from build123d import *

# Parameters (mm, degrees)
SKETCH_1_W          = 19.8
SKETCH_1_H          = 10.2
EXTRUDE_1_DEPTH     = 6.4
SKETCH_2_R          = 1.175
CUT_EXTRUDE_1_DEPTH = 7.4
SKETCH_3_W          = 1
SKETCH_3_H          = 3.2
EXTRUDE_1_2_DEPTH   = 7.7
EXTRUDE_START       = -1
EXTRUDE_2_DEPTH     = 4.4


with BuildPart() as part:
    # 草图1 → Extrude 1 (new body)
    with BuildSketch(Plane.XY):
        Rectangle(SKETCH_1_W, SKETCH_1_H)
    extrude(amount=EXTRUDE_1_DEPTH)

    # 草图2 → 切除-拉伸1 (cut, through all)
    with BuildSketch(Plane(origin=(0, 0, 0), x_dir=(-1, 0, 0), z_dir=(0, 0, -1))):
        with Locations((-4.75, -2.2)):
            Circle(SKETCH_2_R)
        with Locations((4.75, -2.2)):
            Circle(SKETCH_2_R)
    extrude(amount=-CUT_EXTRUDE_1_DEPTH, mode=Mode.SUBTRACT)

    # 草图3 → Extrude 1 2 (add)
    with BuildSketch(Plane(origin=(0, -5.1, 0), x_dir=(-1, 0, 0), z_dir=(0, -1, 0))):
        with Locations((-8.05, -3.2)):
            Rectangle(SKETCH_3_W, SKETCH_3_H)
        with Locations((0.75, -3.2)):
            Rectangle(SKETCH_3_W, SKETCH_3_H)
        with Locations((8.05, -3.2)):
            Rectangle(SKETCH_3_W, SKETCH_3_H)
    extrude(amount=EXTRUDE_1_2_DEPTH)

    # 草图4 → 拉伸-薄壁2 (add)
    with BuildSketch(Plane(origin=(0, 0, 0), x_dir=(-1, 0, 0), z_dir=(0, 0, -1)).offset(EXTRUDE_START)):
        Polygon((-5.054923372, 5.1), (13.203386491, 11.514977847), (13.534867703, 10.571516026), (-4.723442161, 4.15653818), align=None)
    extrude(amount=-EXTRUDE_2_DEPTH)


solid = part.part
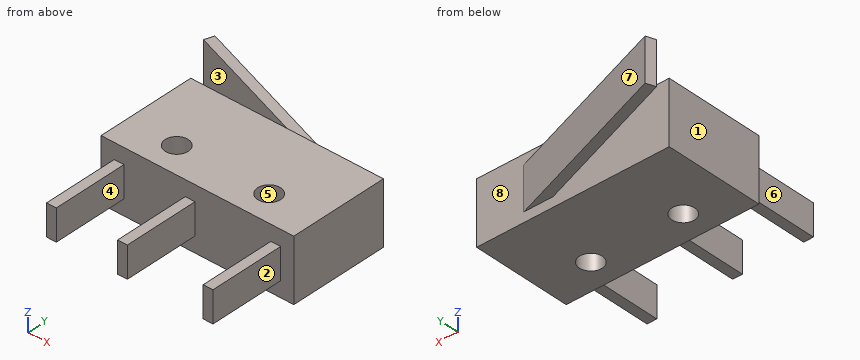
Part model, mm, in its own coordinate system. Face numbers are marked on the shaded views. A direction names the side the tool comes from. Round coordinates to 2 decimals unless told otherwise and drop trailing zeros. Loops run counter-clockwise (first coordinate to the right, second up) from the corner with the lowest first, then second, coordinate; pieces in that order, holes last. Notation, with made-up numbers: (-18, 59.5) - (32, 59.5) arc R19 cw to (32, 88.5) - close; hole circle Ø5 at (0.5, 41.25). An arc over 180 degrees is marked (long way). Answer as a JSON object with one key per item and string values.
Item 1: Pull direction Y, two halves, no side cores. Call the marked faces 6, 7 and 8: pulls with the +Y half, pulls with the -Y half, needs draft (parallel to the pull), parting line crosses it, or undercut.
Output:
{"face 6": "needs draft", "face 7": "pulls with the +Y half", "face 8": "undercut"}
Item 2: Band-saw the part on D-D on x = -8. List the corners of the cut face in (y, z), plus the area to 3 significant figures.
Output:
{"outline": "(-12.8, 1.6) - (-5.1, 1.6) - (-5.1, 0) - (5.1, 0) - (5.1, 6.4) - (-5.1, 6.4) - (-5.1, 4.8) - (-12.8, 4.8) - close; (8.63, 1) - (9.69, 1) - (9.69, 5.4) - (8.63, 5.4) - close", "area": "94.6 mm2"}
Item 3: Wall check: L1, parallel to X at y = -8.75, z = 2; L2, parallel to X at y = -3.75, z = 2.5; L3, parallel to Y at x = -4.75, z = 4.75 (3 decimals). Give the ranges that are in metal, low to high.
Output:
{"L1": "-8.55 to -7.55, -1.25 to -0.25, 7.55 to 8.55", "L2": "-9.9 to 9.9", "L3": "-5.1 to -3.375, -1.025 to 5.1, 7.485 to 8.545"}
Item 4: Band-saw the part on A-A on y = -2.2. List the corners of the cut face in (x, z) (3 decimals).
Output:
{"outline": "(-9.9, 0) - (-5.925, 0) - (-5.925, 6.4) - (-9.9, 6.4) - close; (-3.575, 0) - (3.575, 0) - (3.575, 6.4) - (-3.575, 6.4) - close; (5.925, 0) - (9.9, 0) - (9.9, 6.4) - (5.925, 6.4) - close"}
Item 5: Pin check, flat tips, straight feed: pin 1 (3.5 mm diameter, centred on y = -7.5, z = 3.5, fed in from -X); pin 2 (1.1 mm diameter, centred on x = -0.5, y = -7.5, fed in from +Z); pin 3 (1.6 mm diameter, centred on y = -10, z = 2.5, fed in from +X). Stop position of each tip, or through.
Output:
{"pin 1": "x = -8.55", "pin 2": "z = 4.8", "pin 3": "x = 8.55"}
Item 6: Band-saw the part on C-C on x = -4.75. List the corners of the cut face in (y, z) (3 decimals), plus the area to 3 significant figures.
Output:
{"outline": "(-5.1, 0) - (-3.375, 0) - (-3.375, 6.4) - (-5.1, 6.4) - close; (-1.025, 0) - (5.1, 0) - (5.1, 6.4) - (-1.025, 6.4) - close; (7.485, 1) - (8.545, 1) - (8.545, 5.4) - (7.485, 5.4) - close", "area": "54.9 mm2"}
Item 7: Band-saw the part on B-B on z = 4.25. List the corners of the cut face in (x, y) (3 decimals).
Output:
{"outline": "(-13.535, 10.572) - (2.038, 5.1) - (-9.9, 5.1) - (-9.9, -5.1) - (-8.55, -5.1) - (-8.55, -12.8) - (-7.55, -12.8) - (-7.55, -5.1) - (-1.25, -5.1) - (-1.25, -12.8) - (-0.25, -12.8) - (-0.25, -5.1) - (7.55, -5.1) - (7.55, -12.8) - (8.55, -12.8) - (8.55, -5.1) - (9.9, -5.1) - (9.9, 5.1) - (5.055, 5.1) - (-13.203, 11.515) - close; hole circle Ø2.35 at (-4.75, -2.2); hole circle Ø2.35 at (4.75, -2.2)"}
Item 8: Tool access for the marked faces 1, 2, 3, 4 and 5: list every direction of +Z, -Z, +X, -X, +Y, -Y with a clear straight run to the whole face (end or side of a thin tool).
Output:
{"face 1": "+Z, -Z, -X, -Y", "face 2": "+Z, -Z, +X, -Y", "face 3": "+Z, -Z, -X", "face 4": "+Z, -Z, -Y", "face 5": "+Z, -Z"}
